from build123d import *

# Parameters (mm, degrees)
IZIM1_R                     = 0.8
Y_KSEKLIK_EKSTR_ZYON1_DEPTH = 3
RADYUS1_R                   = 3
KES_EKSTR_ZYON5_REACH       = 83.679
IZIM6_R                     = 0.8


with BuildPart() as part:
    # Çizim1 → Yükseklik-Ekstrüzyon1 (new, symmetric)
    with BuildSketch(Plane.XY):
        with BuildLine():
            Line((-40, 2), (-40, 14.2))
            ThreePointArc((-40, 14.2), (-39.414213562, 15.614213562), (-38, 16.2))
            Line((-38, 16.2), (-36, 16.2))
            Line((-36, 16.2), (-36, 4))
            Line((-36, 4), (-12.8, 4))
            Line((-12.8, 4), (-12.8, 16.2))
            Line((-12.8, 16.2), (-7.8, 16.2))
            Line((-7.8, 16.2), (-5.8, 13.199942957))
            Line((-5.8, 13.199942957), (5.8, 13.199942957))
            Line((5.8, 13.199942957), (7.8, 16.2))
            Line((7.8, 16.2), (11, 16.2))
            Line((11, 16.2), (12.8, 16.2))
            Line((12.8, 16.2), (12.8, 4))
            Line((12.8, 4), (36, 4))
            Line((36, 4), (36, 16.2))
            Line((36, 16.2), (38, 16.2))
            ThreePointArc((38, 16.2), (39.414213562, 15.614213562), (40, 14.2))
            Line((40, 14.2), (40, 2))
            ThreePointArc((40, 2), (39.414213562, 0.585786438), (38, 0))
            Line((38, 0), (9.5, 0))
            Line((9.5, 0), (9.5, 2.199942957))
            ThreePointArc((9.5, 2.199942957), (8.914213562, 3.614156519), (7.5, 4.199942957))
            Line((7.5, 4.199942957), (-7.5, 4.199942957))
            ThreePointArc((-7.5, 4.199942957), (-8.914213562, 3.614156519), (-9.5, 2.199942957))
            Line((-9.5, 2.199942957), (-9.5, 0))
            Line((-9.5, 0), (-38, 0))
            ThreePointArc((-38, 0), (-39.414213562, 0.585786438), (-40, 2))
        make_face()
        with Locations((-10.55, 10.149944348)):
            Circle(IZIM1_R, mode=Mode.SUBTRACT)
        with Locations((-38.25, 10.149944348)):
            Circle(IZIM1_R, mode=Mode.SUBTRACT)
        with Locations(Location((38.25, 10.149944348, 0), (0, 0, 180))):
            Circle(IZIM1_R, mode=Mode.SUBTRACT)
        with Locations(Location((10.55, 10.149944348, 0), (0, 0, 180))):
            Circle(IZIM1_R, mode=Mode.SUBTRACT)
    extrude(amount=Y_KSEKLIK_EKSTR_ZYON1_DEPTH, both=True)

    # Radyus1
    radyus1_edges = [part.edges().sort_by_distance(p)[0] for p in [
        (9.5, 0, 0),
        (-9.5, 0, 0),
    ]]
    fillet(radyus1_edges, radius=RADYUS1_R)

    # Çizim6 → Kes-Ekstrüzyon5 (cut, up to next)
    with BuildSketch(Plane(origin=(40, 0, 0), x_dir=(0, 0, -1), z_dir=(1, 0, 0)), mode=Mode.PRIVATE) as kes_ekstr_zyon5_sk1:
        with Locations((0, 8.1)):
            Circle(IZIM6_R)
    kes_ekstr_zyon5_tool1 = extrude(kes_ekstr_zyon5_sk1.sketch, amount=-KES_EKSTR_ZYON5_REACH, mode=Mode.PRIVATE) & part.part
    add(kes_ekstr_zyon5_tool1.solids().sort_by_distance((40, 8.1, 0))[0], mode=Mode.SUBTRACT)


solid = part.part
Model file for the job. Use its own axes, mm. A direction names the side the tool comes from. Give positions to 0.01 mm unless a question says otherwise; leave off trailing zeros. Loops run counter-clockwise (first coordinate to the right, second up) from the corner with the lowest first, then second, coordinate; pieces in that order, holes last. Notation, with made-up numbers: (-36, 88) -> (16, 88) arc R20 cw to (16, 110) -> close; hole circle Ø9 at (-3.75, 57). An arc over 180 degrees is marked (long way). Use a Markdown table: item, result. Add a question column.
(1) Tool access for faces 4 (the flat face through (-25, 4, 0)), 5 (the cylindrical face through (8.81, 3.71, 0.04)), 6 (the flat face through (-25, 0, 0)): list every direction of +Z, -Z, +X, -X, +Y, -Y with a clear straight run to the whole face (end or side of a thin tool).
(2) Slice it at C-C on x = -25.5. List the corners of the cut face in (y, z), and give its area (3 significant figures).
(3) Slice it at D-D on x = -5. List the corners of the cut face in (y, z), and give its area (3 significant figures).
(4) Mould opens along X. For faces 1 (the flat face through (25, 0, 0)), 2 (the flat face through (-40, 8, 0)), 3 (the flat face through (-7, 15, 0)) say: +X half, -X half, draft (parallel to the pull), parting line (faces both ways), or undercut.
(5) Slice it at A-A on y = 5.75. List the corners of the cut face in (x, z), and give its area (3 significant figures).
(6) Slice it at B-B on z = 0. Give the number of separate pieces and of enclosed holes in the cut face, and give its area (3 significant figures).
(7) Drop flat-ended pins along their axis: pin 1 Ø1.4 at (x, y) = (10.55, 10.15) entering from -Z; pin 2 Ø3 at (x, z) = (-3.5, 0.5) entering from -Y; pin 3 Ø1.5 at (x, z) = (8, -2.5) entering from -Y. Give the stop position or say it passes through.
(8) Wall check: line 1 along X through (y, z) = (6.25, 2.25); line 2 along X through (y, z) = (2.5, -1); line 3 along X through (y, z) = (13.25, -2.25). Give the ranges that are in metal, low to high.
Filled sheet:
| question | item | result |
|---|---|---|
| 1 | face 4 | +Z, -Z, +Y |
| 1 | face 5 | +Z, -Z, -Y |
| 1 | face 6 | +Z, -Z, +X, -X, -Y |
| 2 | outline | (0, -3) -> (4, -3) -> (4, 3) -> (0, 3) -> close |
| 2 | area | 24.0 mm2 |
| 3 | outline | (4.2, -3) -> (13.2, -3) -> (13.2, 3) -> (4.2, 3) -> close |
| 3 | area | 54.0 mm2 |
| 4 | face 1 | draft |
| 4 | face 2 | -X half |
| 4 | face 3 | undercut |
| 5 | outline | (-40, -3) -> (-36, -3) -> (-36, 3) -> (-40, 3) -> close; (-12.8, -3) -> (12.8, -3) -> (12.8, 3) -> (-12.8, 3) -> close; (36, -3) -> (40, -3) -> (40, 3) -> (36, 3) -> close |
| 5 | area | 202 mm2 |
| 6 | separate pieces | 2 |
| 6 | enclosed holes | 4 |
| 6 | area | 590 mm2 |
| 7 | pin 1 | through |
| 7 | pin 2 | y = 4.2 |
| 7 | pin 3 | y = 3.76 |
| 8 | line 1 | -40 to -36, -12.8 to 12.8, 36 to 40 |
| 8 | line 2 | -40 to -9.48, 9.48 to 40 |
| 8 | line 3 | -40 to -36, -12.8 to -5.83, 5.83 to 12.8, 36 to 40 |
